Can you work these out from the model? Positions are in its coordinate system, mm. A direction names the side the tool comes from. Give positions to 0.01 mm unless a question says otherwise; leave off trailing zeros. Write each loop counter-clockwise with the first axis right and the second up, starting at its lowest first coordinate (ties: lowest second). Pieces come first, ordered by that corner, then holes.
1. Suppose I cut it at B-B (z = 0). Please give me the cut outline in (x, y), and give its area (3 significant figures).
2. Thinking about a two-plate mould opening in X: for faces 6 (the cylindrical face through (5.97, 1.23, -7.25)), 7 (the flat face through (0, 15, 8)), 8 (the cylindrical face through (6.03, 1.23, -1.75)), 9 (the flat face through (-6.65, 31, 0)), which applies, pulls with the +X half, pulls with the -X half, needs draft (parallel to the pull), parting line crosses it, or undercut?
3. If I drill on probe 1 along X at (y, z) = (6.5, 0); probe 2 along Y at (x, z) = (3.5, 3.75), over which ranges is the centre line in solid material (lowest first)?
4. On a 3-axis mill with a long thin cutter (end or side, diameter ignored), from which of +Z, -Z, +X, -X, +Y, -Y can I reach the whole of each face in a straight line? I mean faces 1 (the cylindrical face through (-6.01, 30.74, -2.15)), 2 (the cylindrical face through (-5.99, 30.74, 2.15)), 3 (the cylindrical face through (-5.97, 1.23, 7.25)), 4 (the flat face through (0, 15, -8)), 5 (the cylindrical face through (7.4, 14.79, -7.43)). Say none if no direction works.
5. Suppose I cut it at C-C (x = 0). Please give me the cut outline in (y, z), and give its area (3 significant figures).
6. Suppose I cut it at A-A (y = 9). Please give me the cut outline in (x, z), and give its area (3 significant figures).
7. Suppose I cut it at D-D (z = -4). Please give me the cut outline in (x, y) (3 decimals).
8. I'm going to push flat-ended pins straight in: pin 1 (8 mm diameter, centred on x = 0, z = 0, fed in from -Y); pin 2 (1.2 mm diameter, centred on y = 31, z = 0, fed in from +X); pin 3 (5 mm diameter, centred on x = 1, z = -2, fed in from +Y); pin 4 (1.4 mm diameter, centred on x = -6, z = 4.5, fed in from -Y). Where does each tip first touch, or does it pass through?
Autodesk Inventor part; units mm, degrees
ref_plane "YZ Plane" through (0, 0, 0) normal (1, 0, 0) x (0, 1, 0)
ref_plane "XZ Plane" through (0, 0, 0) normal (0, 1, 0) x (-1, 0, 0)
ref_plane "XY Plane" through (0, 0, 0) normal (0, 0, 1) x (1, 0, 0)
sketch "Sketch1" plane through (0, 0, 0) normal (0, 1, 0) x (-1, 0, 0)
  line L0 (6, 8) -> (-6, 8)
  line L1 (-8, 6) -> (-8, -6)
  line L2 (-6, -8) -> (6, -8)
  line L3 (8, -6) -> (8, 6)
  arc A0 (8, 6) -> (6, 8) centre (6, 6) ccw
  arc A1 (-6, 8) -> (-8, 6) centre (-6, 6) ccw
  arc A2 (-8, -6) -> (-6, -8) centre (-6, -6) ccw
  arc A3 (6, -8) -> (8, -6) centre (6, -6) ccw
  point P0 (0, 0)
  point P1 (8, 8)
  point P2 (-8, 8)
  point P3 (8, -8)
  dimension "d0" = 16
  dimension "d1" = 16
  dimension "d2" = 8
  dimension "d3" = 8
  dimension "d4" = 2
extrude "Extrusion1" add sketch "Sketch1" along normal blind 30
sketch "Sketch2" plane through (0, 0, 0) normal (0, -1, 0) x (1, 0, 0)
  line L0 (-6, 5.875) -> (-6, 3.125) construction
  line L1 (-7.375, 5.875) -> (-7.375, 3.125)
  line L2 (-4.625, 3.125) -> (-4.625, 5.875)
  arc A0 (-4.625, 5.875) -> (-7.375, 5.875) centre (-6, 5.875) ccw
  arc A1 (-7.375, 3.125) -> (-4.625, 3.125) centre (-6, 3.125) ccw
  line L3 (6, -3.125) -> (6, -5.875) construction
  line L4 (4.625, -3.125) -> (4.625, -5.875)
  line L5 (7.375, -5.875) -> (7.375, -3.125)
  arc A2 (7.375, -3.125) -> (4.625, -3.125) centre (6, -3.125) ccw
  arc A3 (4.625, -5.875) -> (7.375, -5.875) centre (6, -5.875) ccw
  point P0 (0, 0)
  point P1 (0, 0)
  point P2 (-6, 4.5)
  point P3 (6, -4.5)
  dimension "d7" = 2.75
  dimension "d8" = 12
  dimension "d9" = 6
  dimension "d10" = 9
  dimension "d11" = 4.5
  dimension "d12" = 2.75
  dimension "d13" = 2.75
  dimension "d14" = 2.75
extrude "Extrusion2" cut sketch "Sketch2" against normal blind 2.5
hole "Hole1" at (0, 0, 0) direction (0, 1, 0) diameter 6.756 end through all
sketch "Sketch3" plane through (0, 30, 0) normal (0, 1, 0) x (1, 0, 0)
  line L0 (-6, 1.5) -> (-6, -1.5) construction
  line L1 (-6.65, 1.5) -> (-6.65, -1.5)
  line L2 (-5.35, -1.5) -> (-5.35, 1.5)
  arc A0 (-5.35, 1.5) -> (-6.65, 1.5) centre (-6, 1.5) ccw
  arc A1 (-6.65, -1.5) -> (-5.35, -1.5) centre (-6, -1.5) ccw
  line L3 (6, 1.5) -> (6, -1.5) construction
  line L4 (5.35, 1.5) -> (5.35, -1.5)
  line L5 (6.65, -1.5) -> (6.65, 1.5)
  arc A2 (6.65, 1.5) -> (5.35, 1.5) centre (6, 1.5) ccw
  arc A3 (5.35, -1.5) -> (6.65, -1.5) centre (6, -1.5) ccw
  line L6 (-6, 0) -> (6, 0) construction
  line L7 (6, 8) -> (-6, 8)
  point P0 (0, 0)
  dimension "d25" = 0.65
  dimension "d26" = 0.65
  dimension "d27" = 3
  dimension "d29" = 0
  dimension "d30" = 12
  dimension "d31" = 6
  dimension "d32" = 3
extrude "Extrusion3" add sketch "Sketch3" along normal blind 1.5
equation "\"d12\" = d7"
equation "\"d13\" = d7"
equation "\"d14\" = d7"
equation "\"d26\" = d25"
equation "\"d27\" = d32"
properties part number "Camera Mount 30mm"
Checks:
1. outline: (-8, 0) - (-3.38, 0) - (-3.38, 30) - (-5.35, 30) - (-5.35, 31.5) - (-6.65, 31.5) - (-6.65, 30) - (-8, 30) - close; (3.38, 0) - (8, 0) - (8, 30) - (6.65, 30) - (6.65, 31.5) - (5.35, 31.5) - (5.35, 30) - (3.38, 30) - close
1. area: 281 mm2
2. face 6: undercut
2. face 7: needs draft
2. face 8: undercut
2. face 9: pulls with the -X half
3. probe 1: x = -8 to -3.38, 3.38 to 8
3. probe 2: y = 0 to 30
4. face 1: -Z, +Y
4. face 2: +Z, +Y
4. face 3: -Y
4. face 4: -Z, +X, -X, +Y, -Y
4. face 5: -Z, +X, +Y, -Y
5. outline: (0, -8) - (30, -8) - (30, -3.38) - (0, -3.38) - close; (0, 3.38) - (30, 3.38) - (30, 8) - (0, 8) - close
5. area: 277 mm2
6. outline: (-8, -6) arc R2 ccw to (-6, -8) - (6, -8) arc R2 ccw to (8, -6) - (8, 6) arc R2 ccw to (6, 8) - (-6, 8) arc R2 ccw to (-8, 6) - close; hole circle Ø6.76 at (0, 0)
6. area: 217 mm2
7. outline: (-8, 0) - (4.625, 0) - (4.625, 2.5) - (7.375, 2.5) - (7.375, 0) - (8, 0) - (8, 30) - (-8, 30) - close
8. pin 1: stops at y = 0
8. pin 2: stops at x = 6.65
8. pin 3: stops at y = 30
8. pin 4: stops at y = 2.5
